from build123d import *

# Parameters (mm, degrees)
SKETCH_1_W                = 20.000000045
SKETCH_1_H                = 28
EXTRUDE_1_DEPTH           = 10.000000062
HOLE_WIZARD_5_0_5_1_D     = 5
HOLE_WIZARD_5_0_5_2_D     = 5
HOLE_WIZARD_4_0_4_1_D     = 4
HOLE_WIZARD_4_0_4_1_DEPTH = 40.5
CHAMFER_1_SIZE            = 3.000000071
CHAMFER_1_SIZE2           = 6.000000142


with BuildPart() as part:
    # 草图1 → 凸台-拉伸1 (new body)
    with BuildSketch(Plane(origin=(0, -65.00000108, 0), x_dir=(1, 0, 0), z_dir=(0, 1, 0))):
        with Locations((59.999999934, 33.500000026)):
            Rectangle(SKETCH_1_W, SKETCH_1_H)
    extrude(amount=-EXTRUDE_1_DEPTH)

    # Ø5.0 (5) 直径孔1 (through all)
    with Locations(Plane(origin=(0, -75.000001142, 0), x_dir=(-1, 0, 0), z_dir=(0, -1, 0))):
        with Locations((-55.999998876, 25.500000109), (-55.999998876, 41.500000109)):
            Hole(HOLE_WIZARD_5_0_5_1_D / 2)

    # Ø5.0 (5) 直径孔2 (through all)
    with Locations(Plane.ZY.offset(-49.999999911)):
        with Locations((-33.500000026, -70.000000195)):
            Hole(HOLE_WIZARD_5_0_5_2_D / 2)

    # Ø4.0 (4) 直径孔1
    with Locations(Plane(origin=(0, 0, -47.500000026), x_dir=(-1, 0, 0), z_dir=(0, 0, -1))):
        with Locations((-61, -70)):
            Hole(HOLE_WIZARD_4_0_4_1_D / 2, depth=HOLE_WIZARD_4_0_4_1_DEPTH)

    # 倒角1
    chamfer_1_edges = [part.edges().sort_by_distance(p)[0] for p in [
        (49.999999911, -70.000001111, -47.500000026),
        (49.999999911, -70.000001111, -19.500000026),
    ]]
    chamfer_1_side = [part.faces().sort_by_distance(p)[0] for p in [
        (49.999999911, -70.000001111, -47.202678651),
    ]]
    chamfer(chamfer_1_edges, length=CHAMFER_1_SIZE, length2=CHAMFER_1_SIZE2, reference=chamfer_1_side[0])


solid = part.part
Design review of the part built by this model. Coordinates are the model's own, in mm. Coordinates: 2 decimals unless noted, no trailing zeros. Loops run counter-clockwise (first coordinate to the right, second up) from the corner with the lowest first, then second, coordinate; pieces in that order, holes last.
Item 1: Add section B-B (x = 61). Write out the cut boundary in (y, z), and give its area (3 significant figures).
Completed:
outline: (-75, -47.5) - (-72, -47.5) - (-72, -35) arc R2.5 cw to (-72, -32) - (-72, -19.5) - (-75, -19.5) - close; (-68, -47.5) - (-65, -47.5) - (-65, -19.5) - (-68, -19.5) - (-68, -32) arc R2.5 cw to (-68, -35) - close
area: 166 mm2
Item 2: Wall thickness on L1, parallel to X at y = -70, z = -25.5; L2, parallel to X at y = -70, z = -37.5; L3, parallel to Y at x = 61, z = -23.5: over which ranges is each line inside the solid? List them lowest first.
Completed:
L1: x = 50 to 53.5, 58.5 to 59, 63 to 70
L2: x = 50 to 59, 63 to 70
L3: y = -75 to -72, -68 to -65
Item 3: Add section C-C (y = -70). Write out the cut boundary in (x, z).
Completed:
outline: (50, -44.5) - (56, -47.5) - (59, -47.5) - (59, -36) - (50, -36) - close; (50, -31) - (59, -31) - (59, -19.5) - (56, -19.5) - (50, -22.5) - close; (63, -47.5) - (70, -47.5) - (70, -36) - (63, -36) - close; (63, -31) - (70, -31) - (70, -19.5) - (63, -19.5) - close; hole circle Ø5 at (56, -41.5); hole circle Ø5 at (56, -25.5)
Item 4: Add section D-D (x = 56.5). Write out the cut boundary in (y, z).
Completed:
outline: (-75, -47.5) - (-65, -47.5) - (-65, -43.95) - (-75, -43.95) - close; (-75, -39.05) - (-65, -39.05) - (-65, -27.95) - (-75, -27.95) - close; (-75, -23.05) - (-65, -23.05) - (-65, -19.5) - (-75, -19.5) - close; hole circle Ø5 at (-70, -33.5)
Item 5: Draft analysis for pull direction Y (two halves, no side actions). For faces 1 (the flat face through (63, -69, -19.5)), 2 (the cylindrical face through (59, -70, -26)), 3 (the flat face through (60, -65, -34)), state which applies: pulls with the +Y half, pulls with the -Y half, needs draft (parallel to the pull), parting line crosses it, or undercut.
Completed:
face 1: needs draft
face 2: undercut
face 3: pulls with the +Y half
Item 6: Add section A-A (z = -39.5). Write out the cut boundary in (x, y).
Completed:
outline: (50, -75) - (54.5, -75) - (54.5, -65) - (50, -65) - close; (57.5, -75) - (70, -75) - (70, -65) - (57.5, -65) - close; hole circle Ø4 at (61, -70)
